```python
from build123d import *

# Parameters (mm, degrees)
ESBO_O3_W                = 16
ESBO_O3_H                = 16
RESSALTO_EXTRUS_O1_DEPTH = 12
ESBO_O4_R                = 3
RESSALTO_EXTRUS_O2_DEPTH = 5
RESSALTO_EXTRUS_O2_TAPER = 26


with BuildPart() as part:
    # Esboço1 → Revolução1 (revolve)
    with BuildSketch(Plane.XY, mode=Mode.PRIVATE) as revolu_o1_sk:
        Polygon((0, 51.659238703), (0, 1.659238703), (2, 1.659238703), (2, 2.659238703), (12.35, 2.659238703), (12.35, 3.659238703), (4, 3.659238703), (4, 6.103683147), (12.35, 6.103683147), (12.35, 7.103683147), (4, 7.103683147), (4, 9.548127592), (12.35, 9.548127592), (12.35, 10.548127592), (4, 10.548127592), (4, 12.992572036), (12.35, 12.992572036), (12.35, 13.992572036), (4, 13.992572036), (4, 16.437016481), (12.35, 16.437016481), (12.35, 17.437016481), (4, 17.437016481), (4, 19.881460925), (12.35, 19.881460925), (12.35, 20.881460925), (4, 20.881460925), (4, 23.32590537), (12.35, 23.32590537), (12.35, 24.32590537), (4, 24.32590537), (4, 26.770349814), (12.35, 26.770349814), (12.35, 27.770349814), (4, 27.770349814), (4, 30.214794259), (12.35, 30.214794259), (12.35, 31.214794259), (4, 31.214794259), (4, 33.659238703), (12.35, 33.659238703), (12.35, 34.659238703), (4, 34.659238703), (4, 39.959238703), (8, 39.959238703), (8, 42.659238703), (5.5, 42.659238703), (5.5, 48.159238703), (8, 48.159238703), (8, 51.659238703), align=None)
    revolve(revolu_o1_sk.sketch.rotate(Axis((0, 51.659238703, 0), (0, -1, 0)), 180), axis=Axis((0, 51.659238703, 0), (0, -1, 0)))

    # Esboço3 → Ressalto-extrusão1 (add)
    with BuildSketch(Plane.XZ.offset(-1.659238703)):
        with Locations((0, 4)):
            Rectangle(ESBO_O3_W, ESBO_O3_H)
    extrude(amount=RESSALTO_EXTRUS_O1_DEPTH)

    # Esboço4 → Ressalto-extrusão2 (add)
    with BuildSketch(Plane.XZ.offset(10.340761297)):
        Circle(ESBO_O4_R)
    extrude(amount=RESSALTO_EXTRUS_O2_DEPTH, taper=RESSALTO_EXTRUS_O2_TAPER)


solid = part.part
```
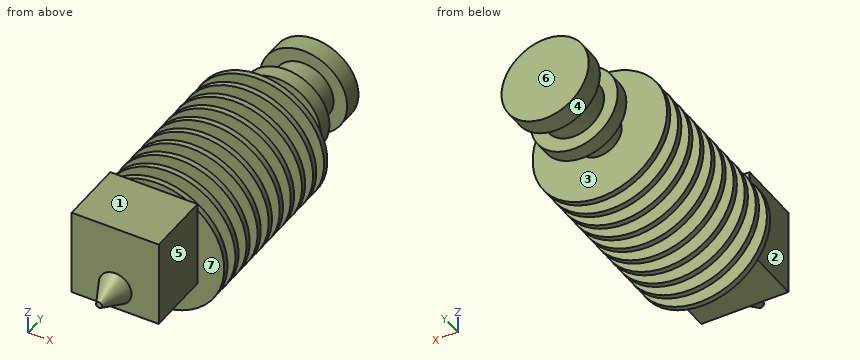
Input: part model. Units: mm. Frame: model coordinates. Face numbers are marked on the shaded views. A direction names the side the tool comes from. Coordinates: 2 decimals unless noted, no trailing zeros. Order: outer loops, then holes, each group sorted by start corner. A loop starts at its lowest first (then second) coordinate and runs counter-clockwise, first axis right, second up. Notation, with made-up numbers: (-35, -3.75) - (-31, -3.75) arc R32 cw to (-31, 28.25) - close; hole circle Ø4 at (11.5, 57.5). An arc over 180 degrees is marked (long way). Return JSON: item names as keys, results as strings.
Q1. Ray query, probe 1 along Y at (x, z) = (2.75, 1.5); probe 2 along Z at (x, y) = (-1.5, 1); probe 3 along X at (y, z) = (-2, 6). Return the intervals inside material, ascending.
The answers:
{"probe 1": "y = -10.34 to 1.66, 2.66 to 51.66", "probe 2": "z = -4 to 12", "probe 3": "x = -8 to 8"}
Q2. Access query for the marked faces 1, 2, 3 and 4. Directions: +Z, -Z, +X, -X, +Y, -Y. A direction counts if a zero-diameter tool reaches every point of the face in a straight line with its end or side. Return the directions, or none.
The answers:
{"face 1": "+Z, +X, -X, -Y", "face 2": "+Z, -Z, -X, -Y", "face 3": "none", "face 4": "+Y"}
Q3. Cut plane A-A (y = 38). Return loops of the section in (x, z), then the cut area to 3 significant figures.
The answers:
{"outline": "circle Ø8 at (0, 0)", "area": "50.3 mm2"}
Q4. First-contact query: pin 1 (12 mm diameter, centred on y = -5, z = 2, fed in from +X); pin 2 (5 mm diameter, centred on x = 1.5, z = -8, fed in from -Y); pin 3 (10 mm diameter, centred on x = -8, y = 34, fed in from +Z); pin 4 (8 mm diameter, centred on y = 7.5, z = 2.5, fed in from +X). Flat tips, straight axial feed; report the tip coordinate or a pass-through.
The answers:
{"pin 1": "stops at x = 8", "pin 2": "stops at y = 2.66", "pin 3": "stops at z = 11.98", "pin 4": "stops at x = 12.35"}
Q5. Cut plane B-B (z = -6.25). State how many separate pieces and enclosed holes the cut face has, then the cut area to 3 significant figures.
The answers:
{"separate pieces": "12", "enclosed holes": "0", "area": "275 mm2"}
Q6. Draft query along Y for the marked faces 5, 6 and 7. Return one class per face: +Y half, -Y half, draft (parallel to the pull), parting line (faces both ways), or undercut.
The answers:
{"face 5": "draft", "face 6": "+Y half", "face 7": "undercut"}
